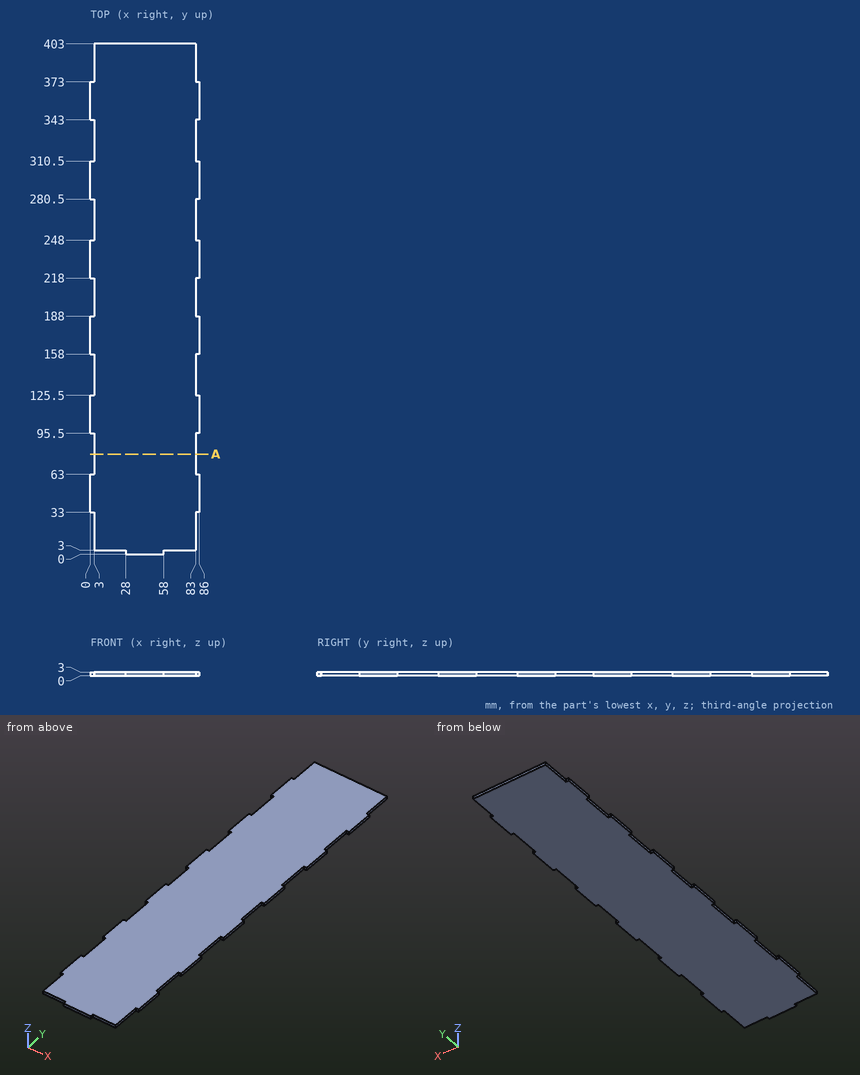
The figure shows three views and two pictorial views of one solid part (mm, origin at its lowest corner). Answer the questions. Round coordinates to 2 decimals unless told otherwise and drop trailing zeros. Write each loop counter-clockwise with the first axis right and the second up, starting at its lowest first coordinate (ties: lowest second). Pieces come first, ordered by that corner, then holes. Notation, with made-up numbers: (-17, 71) -> (18, 71) arc R4 ccw to (18, 76) -> close; hole circle Ø3 at (80, -38.5). An arc over 180 degrees is marked (long way). Write each question's results on one line, items separated by ' | '.
Q1. Straight lines are drawn through the part: line 1 along Y through (x, z) = (64, 0.65); line 2 along X through (y, z) = (128.5, 0.3). For each, find the intervals that lie inside material, in ascending order. Write a range as [from, to].
Data:
line 1: [3, 403] | line 2: [3, 83]
Q2. Section A-A, the plane y = 79 is taken. Write down the section's boundary in (x, z).
Data:
outline: (3, 0) -> (83, 0) -> (83, 3) -> (3, 3) -> close
Q3. Flat-ended cylindrical pins translate along their axes: P1, Ø1.5, axis at x = 2, z = 1.5, coming from the -Y side; P2, Ø1.5, axis at x = 2, z = 1, coming from the +Y side; P3, Ø10, axis at x = 11, y = 149.5, coming from the -Z side; P4, Ø0.9, axis at y = 325.5, z = 1, coming from the -X side. Find the tip coordinate at first contact, or state that the pin passes through.
Data:
P1: y = 33 | P2: y = 373 | P3: z = 0 | P4: x = 3
